from build123d import *

# Parameters (mm, degrees)
BOSS_EXTRUDE1_DEPTH              = 3.81
TAP_DRILL_FOR_5_16_18_TAP1_D     = 6.5278
TAP_DRILL_FOR_5_16_18_TAP1_DEPTH = 25.4
TAP_DRILL_FOR_5_16_18_TAP1_TIP   = 1.961148974


with BuildPart() as part:
    # Sketch1 → Boss-Extrude1 (new body)
    with BuildSketch(Plane(origin=(0, 0, 0), x_dir=(0, 1, 0), z_dir=(0, 0, 1))):
        Polygon((0, -7.332348419), (6.35, -3.666174209), (6.35, 3.666174209), (0, 7.332348419), (-6.35, 3.666174209), (-6.35, -3.666174209), align=None)
    extrude(amount=BOSS_EXTRUDE1_DEPTH)

    # Tap Drill for 5/16-18 Tap1
    with Locations(Plane.XY.offset(3.81)):
        with Locations((0, 0)):
            Hole(TAP_DRILL_FOR_5_16_18_TAP1_D / 2, depth=TAP_DRILL_FOR_5_16_18_TAP1_DEPTH)
            with Locations((0, 0, -(TAP_DRILL_FOR_5_16_18_TAP1_DEPTH + TAP_DRILL_FOR_5_16_18_TAP1_TIP / 2))):  # 118° drill point
                Cone(0, TAP_DRILL_FOR_5_16_18_TAP1_D / 2, TAP_DRILL_FOR_5_16_18_TAP1_TIP, mode=Mode.SUBTRACT)


solid = part.part
Could you check a few things on this model? Use its own coordinates, in mm. Give positions to 0.01 mm unless a question says otherwise; leave off trailing zeros. Order: outer loops, then holes, each group sorted by start corner. A loop starts at its lowest first (then second) coordinate and runs counter-clockwise, first axis right, second up. Notation, with made-up numbers: (85, 60) -> (142, 60) arc R15 ccw to (142, 79) -> close; hole circle Ø11 at (4.25, -3). An arc over 180 degrees is marked (long way). Answer in a Markdown table with one row per item. Add a question column.
Item 1: Imagine slicing it at A-A (x = 3). List the corners of the cut face in (y, z) for me.
Item 2: Imagine slicing it at B-B (y = -0.5). List the corners of the cut face in (x, z) for me.
Item 3: Imagine slicing it at D-D (x = -4.5). List the corners of the cut face in (y, z) for me, and give its area (3 significant figures).
Item 4: I'm going to push a flat-ended pin straight in: P1, Ø6, axis at x = 0, y = 0, coming from the +Z side. Where does the tip first touch, or does it pass through?
Item 5: We'd pull the mould along X, two halves only. Please class faces 1 (the flat face through (5.525, 3.131, 1.878)), 2 (the flat face through (2, -3, 3.81)), 3 (the cylindrical face through (0.708, -3.186, 1.878)), 4 (the flat face through (-5.525, -3.131, 1.878)): pulls with the +X half, pulls with the -X half, needs draft (parallel to the pull), parting line crosses it, or undercut.
Item 6: Please list where these lines run through material, in increasing order: probe 1 along Y at (x, z) = (0, 1.25); probe 2 along X at (y, z) = (-1.75, 1.25); probe 3 along Y at (x, z) = (1.5, 1.65).
Item 7: Imagine slicing it at C-C (z = 2.4). List the corners of the cut face in (x, y) for me, and give its area (3 significant figures).
Result:
| question | item | result |
|---|---|---|
| 1 | outline | (-6.35, 0) -> (-1.29, 0) -> (-1.29, 3.81) -> (-6.35, 3.81) -> close; (1.29, 0) -> (6.35, 0) -> (6.35, 3.81) -> (1.29, 3.81) -> close |
| 2 | outline | (-7.04, 0) -> (-3.23, 0) -> (-3.23, 3.81) -> (-7.04, 3.81) -> close; (3.23, 0) -> (7.04, 0) -> (7.04, 3.81) -> (3.23, 3.81) -> close |
| 3 | outline | (-4.91, 0) -> (4.91, 0) -> (4.91, 3.81) -> (-4.91, 3.81) -> close |
| 3 | area | 37.4 mm2 |
| 4 | P1 | through |
| 5 | face 1 | pulls with the +X half |
| 5 | face 2 | needs draft |
| 5 | face 3 | undercut |
| 5 | face 4 | pulls with the -X half |
| 6 | probe 1 | -6.35 to -3.26, 3.26 to 6.35 |
| 6 | probe 2 | -6.32 to -2.76, 2.76 to 6.32 |
| 6 | probe 3 | -6.35 to -2.9, 2.9 to 6.35 |
| 7 | outline | (-7.33, 0) -> (-3.67, -6.35) -> (3.67, -6.35) -> (7.33, 0) -> (3.67, 6.35) -> (-3.67, 6.35) -> close; hole circle Ø6.53 at (0, 0) |
| 7 | area | 106 mm2 |
